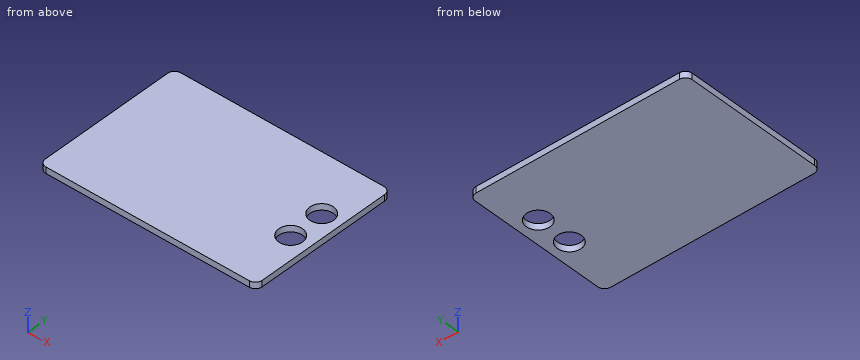
```python
from build123d import *

# Parameters (mm, degrees)
F0_W     = 82
F0_H     = 56.95
F1_DEPTH = 2.35
F2_R     = 2.54
F3_R     = 4.5
F4_DEPTH = 2.35


with BuildPart() as f1:
    # F0 (on Top) → F1 (new body)
    with BuildSketch(Plane.XY):
        Rectangle(F0_W, F0_H)
    extrude(amount=F1_DEPTH)

    # F2
    f2_edges = [f1.edges().sort_by_distance(p)[0] for p in [
        (-41, 28.475, 1.175),
        (-41, -28.475, 1.175),
        (41, 28.475, 1.175),
        (41, -28.475, 1.175),
    ]]
    fillet(f2_edges, radius=F2_R)

    # F3 (on face) → F4 (cut, through all)
    with BuildSketch(Plane.XY.offset(2.35)):
        with Locations((33.5, 7.675)):
            Circle(F3_R)
        with Locations((33.5, -5.475)):
            Circle(F3_R)
    extrude(amount=-F4_DEPTH, mode=Mode.SUBTRACT)


solid = f1.part
```
For this review, take the finished solid that the model builds, in its own axes (mm). Coordinates: 2 decimals unless noted, no trailing zeros. Write each loop counter-clockwise with the first axis right and the second up, starting at its lowest first coordinate (ties: lowest second). Pieces come first, ordered by that corner, then holes. Notation, with made-up numbers: (64, -30.75) - (92, -30.75) arc R11 ccw to (92, -17.75) - close; hole circle Ø10 at (-37.5, -11). An arc over 180 degrees is marked (long way). Put each result on its own line as item: value.
1. Add section C-C, the plane z = 1.75. Give the boundary of the cut face in (x, y) (3 decimals), then the cut area to 3 significant figures.
Values found:
outline: (-41, -25.935) arc R2.54 ccw to (-38.46, -28.475) - (38.46, -28.475) arc R2.54 ccw to (41, -25.935) - (41, 25.935) arc R2.54 ccw to (38.46, 28.475) - (-38.46, 28.475) arc R2.54 ccw to (-41, 25.935) - close; hole circle Ø9 at (33.5, -5.475); hole circle Ø9 at (33.5, 7.675)
area: 4,540 mm²
2. Wall thickness on probe 1 along Y at (x, z) = (33.5, 1.35) (3 decimals); probe 2 along Y at (x, z) = (36.5, 1.6) (3 decimals); probe 3 along X at (y, z) = (9, 0.7): over which ranges is each line inside the solid? List them lowest first.
Values found:
probe 1: -28.475 to -9.975, -0.975 to 3.175, 12.175 to 28.475
probe 2: -28.475 to -8.829, -2.121 to 4.321, 11.029 to 28.475
probe 3: -41 to 29.2, 37.8 to 41
3. Add section A-A, the plane x = 33.5. Give the boundary of the cut face in (y, z) (3 decimals).
Values found:
outline: (-28.475, 0) - (-9.975, 0) - (-9.975, 2.35) - (-28.475, 2.35) - close; (-0.975, 0) - (3.175, 0) - (3.175, 2.35) - (-0.975, 2.35) - close; (12.175, 0) - (28.475, 0) - (28.475, 2.35) - (12.175, 2.35) - close
4. Add section D-D, the plane y = -9. Give the boundary of the cut face in (x, z).
Values found:
outline: (-41, 0) - (30.7, 0) - (30.7, 2.35) - (-41, 2.35) - close; (36.3, 0) - (41, 0) - (41, 2.35) - (36.3, 2.35) - close
5. Add section B-B, the plane y = 4.5. Give the boundary of the cut face in (x, z), then the cut area to 3 significant figures.
Values found:
outline: (-41, 0) - (30.31, 0) - (30.31, 2.35) - (-41, 2.35) - close; (36.69, 0) - (41, 0) - (41, 2.35) - (36.69, 2.35) - close
area: 178 mm²
